Could you check a few things on this model? Use its own coordinates, in mm. A direction names the side the tool comes from. Round coordinates to 2 decimals unless told otherwise and drop trailing zeros. Order: outer loops, then holes, each group sorted by start corner. A loop starts at its lowest first (then second) coordinate and runs counter-clockwise, first axis right, second up. Notation, with made-up numbers: (73.5, 82.25) - (100.5, 82.25) arc R34 ccw to (100.5, 119.25) - close; hole circle Ø4 at (58, -7). An arc over 180 degrees is marked (long way). Return JSON: item names as keys, results as strings. Group by question number.
from build123d import *

# Parameters (mm, degrees)
CROQUIS2_W                  = 37
CROQUIS2_H                  = 20
SALIENTE_EXTRUIR2_DEPTH     = 20
CORTAR_EXTRUIR2_DEPTH       = 47.572524089
CORTAR_EXTRUIR2_DEPTH_BACK  = 47.572524089
CROQUIS3_W                  = 15
CROQUIS3_H                  = 10
CROQUIS4_R                  = 3
CORTAR_EXTRUIR3_DEPTH       = 44.231932642
CROQUIS8_W                  = 15
CROQUIS8_H                  = 20
SALIENTE_EXTRUIR4_DEPTH     = 2.679491924
CORTAR_EXTRUIR10_DEPTH      = 36.832945734
CORTAR_EXTRUIR10_DEPTH_BACK = 36.832945734
MOVER_START                 = -20
MOVER_CARA2_DEPTH           = 10
MOVER_START_2               = -10
MOVER_CARA2_2_OUTLINE_W     = 22
MOVER_CARA2_2_OUTLINE_H     = 2.679491924
MOVER_CARA2_2_OUTLINE_R     = 3
MOVER_CARA2_2_DEPTH         = 10
MOVER_CARA2_3_OUTLINE_R     = 3
MOVER_CARA2_3_DEPTH         = 10
MOVER_CARA2_4_OUTLINE_W     = 22
MOVER_CARA2_4_OUTLINE_H     = 2.679491924
MOVER_CARA2_4_OUTLINE_R     = 3
MOVER_CARA2_4_DEPTH         = 10
MOVER_CARA2_5_DEPTH         = 15
MOVER_CARA2_6_DEPTH         = 15


with BuildPart() as part:
    # Croquis2 → Saliente-Extruir2 (new body)
    with BuildSketch(Plane(origin=(0, 0, 0), x_dir=(1, 0, 0), z_dir=(0, 1, 0))):
        with Locations((18.5, 10)):
            Rectangle(CROQUIS2_W, CROQUIS2_H)
    extrude(amount=SALIENTE_EXTRUIR2_DEPTH)

    # Croquis3 → Cortar-Extruir2 (cut, two sides: drawn at the far end of the back side and taken through both)
    with BuildSketch(Plane(origin=(0, 0, 0), x_dir=(1, 0, 0), z_dir=(0, 1, 0)).offset(-CORTAR_EXTRUIR2_DEPTH_BACK)):
        with Locations((7.5, 15)):
            Rectangle(CROQUIS3_W, CROQUIS3_H)
    extrude(amount=CORTAR_EXTRUIR2_DEPTH + CORTAR_EXTRUIR2_DEPTH_BACK, mode=Mode.SUBTRACT)

    # Croquis4 → Cortar-Extruir3 (cut, through all)
    with BuildSketch(Plane(origin=(0, 0, -10), x_dir=(-1, 0, 0), z_dir=(0, 0, -1))):
        with Locations((-7.5, 10)):
            Circle(CROQUIS4_R)
    extrude(amount=-CORTAR_EXTRUIR3_DEPTH, mode=Mode.SUBTRACT)

    # Croquis8 → Saliente-Extruir4 (add)
    with BuildSketch(Plane.XZ):
        with Locations((29.5, -10)):
            Rectangle(CROQUIS8_W, CROQUIS8_H)
    extrude(amount=SALIENTE_EXTRUIR4_DEPTH)

    # Croquis9 → Cortar-Extruir10 (cut, two sides: drawn at the far end of the back side and taken through both)
    with BuildSketch(Plane.ZY.offset(-22).offset(-CORTAR_EXTRUIR10_DEPTH_BACK)):
        with BuildLine():
            Line((-81.034656774, -37.917867438), (-20, -2.679491924))
            ThreePointArc((-20, -2.679491924), (-10, 0), (0, -2.679491924))
            Line((0, -2.679491924), (61.034656774, -37.917867438))
            Line((61.034656774, -37.917867438), (61.034656774, -178.871369507))
            Line((61.034656774, -178.871369507), (-81.034656774, -178.871369507))
            Line((-81.034656774, -178.871369507), (-81.034656774, -37.917867438))
        make_face()
    extrude(amount=CORTAR_EXTRUIR10_DEPTH + CORTAR_EXTRUIR10_DEPTH_BACK, mode=Mode.SUBTRACT)

    # Mover cara2: read off the stored shape, not the designer's step
    # Mover cara2 outline → Mover cara2 (cut)
    with BuildSketch(Plane.XY.offset(MOVER_START)):
        Polygon((15, 20), (15, 17.320508076), (22, 17.320508076), (22, -2.679491924), (37, -2.679491924), (37, 20), align=None)
    extrude(amount=MOVER_CARA2_DEPTH, mode=Mode.SUBTRACT)

    # Mover cara2 2 outline → Mover cara2 2 (cut)
    with BuildSketch(Plane.XY.offset(MOVER_START_2)):
        with Locations((26, 18.660254038)):
            Rectangle(MOVER_CARA2_2_OUTLINE_W, MOVER_CARA2_2_OUTLINE_H)
        with Locations((29.5, 7.320508076)):
            Circle(MOVER_CARA2_2_OUTLINE_R)
    extrude(amount=MOVER_CARA2_2_DEPTH, mode=Mode.SUBTRACT)

    # Mover cara2 3 outline → Mover cara2 3 (add)
    # profile 1 of 2: a face of its own
    with BuildSketch(Plane.XY.offset(MOVER_START_2)):
        Polygon((37, 17.320508076), (22, 17.320508076), (22, 0), (0, 0), (0, -2.679491924), (37, -2.679491924), align=None)
        with Locations((29.5, 7.320508076)):
            Circle(MOVER_CARA2_3_OUTLINE_R, mode=Mode.SUBTRACT)
    # profile 2 of 2: a face of its own
    with BuildSketch(Plane.XY.offset(MOVER_START_2)):
        with Locations((7.5, 10)):
            Circle(MOVER_CARA2_3_OUTLINE_R)
    extrude(amount=MOVER_CARA2_3_DEPTH)

    # Mover cara2 4 outline → Mover cara2 4 (add)
    with BuildSketch(Plane.XY.offset(MOVER_START)):
        with Locations((11, -1.339745962)):
            Rectangle(MOVER_CARA2_4_OUTLINE_W, MOVER_CARA2_4_OUTLINE_H)
        with Locations((7.5, 10)):
            Circle(MOVER_CARA2_4_OUTLINE_R)
    extrude(amount=MOVER_CARA2_4_DEPTH)

    # Mover cara2 5 outline → Mover cara2 5 (cut)
    with BuildSketch(Plane.YZ):
        with BuildLine():
            ThreePointArc((20, 0), (18.00199155, -4.823619098), (17.320508076, -10))
            Line((17.320508076, -10), (20, -10))
            Line((20, -10), (20, 0))
        make_face()
    extrude(amount=MOVER_CARA2_5_DEPTH, mode=Mode.SUBTRACT)

    # Mover cara2 6 outline → Mover cara2 6 (add)
    with BuildSketch(Plane.YZ):
        with BuildLine():
            Line((0, -20), (20, -20))
            ThreePointArc((20, -20), (18.00199155, -15.176380902), (17.320508076, -10))
            Line((17.320508076, -10), (0, -10))
            Line((0, -10), (0, -20))
        make_face()
    extrude(amount=MOVER_CARA2_6_DEPTH)


solid = part.part
1) We'd pull the mould along Y, two halves only. Please class faces 1 (the flat face through (14, -2.679, -8)), 2 (the cylindrical face through (26.503, 7.452, -5.07)), 3 (the flat face through (23, 17.321, -8)): +Y half, -Y half, draft (parallel to the pull), parting line (faces both ways), or undercut.
2) For faces 4 (the flat face through (26, 7, -10)), 5 (the flat face through (18, 9, 0)), 6 (the flat face through (15, 18, -18)), which set-ups out of +Z, -Z, +X, -X, +Y, -Y let a thin tool reach every point of the face, with its end or its side?
3) I want a section at B-B, the plane x = 29.5. List the corners of the cut face in (y, z) for me.
4) If I drill on line 1 along Y through (x, z) = (29.5, -3.5); line 2 along Y through (x, z) = (6.5, -9.5); line 3 along Z through (x, y) = (26, -0.5), over which ranges is the centre line in solid material (lowest first)? Write a range as from..to.
5) Will these pins go through, and if not, where does the flat tip stop? pin 1 (3 mm diameter, centred on y = 19, z = -14, fed in from +X); pin 2 (1 mm diameter, centred on x = 18, z = -4.5, fed in from +Y); pin 3 (3.5 mm diameter, centred on x = 29.5, y = 7.32, fed in from +Z); pin 4 (5 mm diameter, centred on x = 26.5, y = 8.5, fed in from -Z).
6) I want a section at D-D, the plane x = 8. List the corners of the cut face in (y, z) for me.
7) I want a section at A-A, the plane y = 5.5. List the corners of the cut face in (x, z) for me.
8) I want a section at C-C, the plane z = -5.75. List the corners of the cut face in (x, y) for me.
Outcome:
{
 "1": {"face 1": "-Y half", "face 2": "undercut", "face 3": "+Y half"},
 "2": {"face 4": "-Z, +X, +Y, -Y", "face 5": "+Z, +X, -X, +Y, -Y", "face 6": "+Z, -Z, +X, +Y"},
 "3": {"outline": "(-2.68, -10) - (4.32, -10) - (4.32, 0) - (-2.68, 0) - close; (10.32, -10) - (17.32, -10) - (17.32, 0) - (10.32, 0) - close"},
 "4": {"line 1": "-2.68..4.32, 10.32..17.32", "line 2": "-2.68..17.33", "line 3": "-10..0"},
 "5": {"pin 1": "x = 15", "pin 2": "y = 17.32", "pin 3": "through", "pin 4": "z = -10"},
 "6": {"outline": "(-2.68, -20) - (20, -20) arc R20 cw to (20, 0) - (-2.68, 0) - close"},
 "7": {"outline": "(0, -20) - (22, -20) - (22, -10) - (27.12, -10) - (27.12, 0) - (0, 0) - close; (31.88, -10) - (37, -10) - (37, 0) - (31.88, 0) - close"},
 "8": {"outline": "(0, -2.68) - (37, -2.68) - (37, 17.32) - (15, 17.32) - (15, 17.78) - (0, 17.78) - close; hole circle Ø6 at (29.5, 7.32)"}
}
